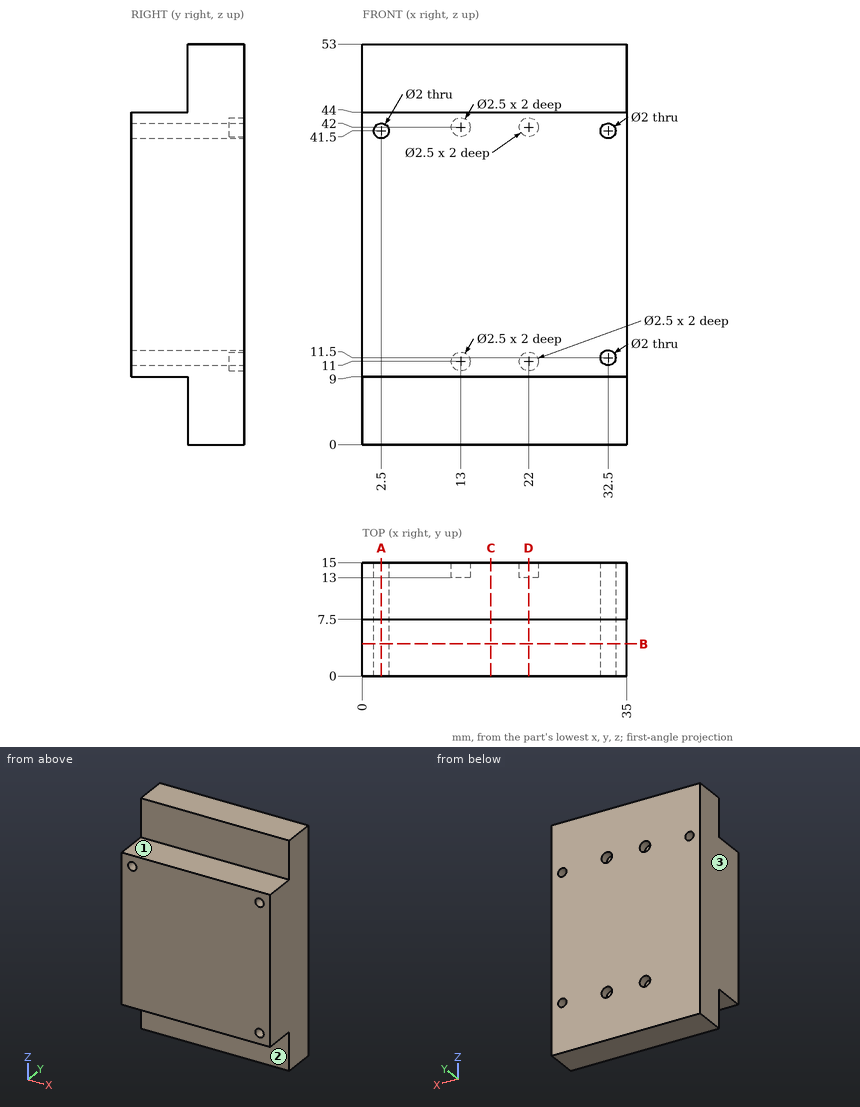
For this review, use the dimensioned drawing (mm, ordinates from the lowest corner) and the shaded views. A direction names the side the tool comes from. Give positions to 0.01 mm unless a question says otherwise; leave off trailing zeros. Write each loop counter-clockwise with the first axis right and the second up, starting at its lowest first coordinate (ties: lowest second). Pieces come first, ordered by that corner, then holes.
(1) Consider section A-A, the plane x = 2.5. Give the boundary of the cut face in (y, z), and give its area (3 significant figures).
(2) Consider section C-C, the plane x = 17. Give the boundary of the cut face in (y, z).
(3) Tool access review of the marked faces 1, 2 and 3: name each direction out of +Z, -Z, +X, -X, +Y, -Y from which nothing blocks a thin tool from reaching the whole face with its end or side.
(4) Consider section B-B, the plane y = 4.25. Give the boundary of the cut face in (x, z).
(5) To check wall thickness, follow L1, parallel to Z at x = 32.5, y = 3.75; L2, parallel to Z at x = 22, y = 14; L3, parallel to X at y = 14.5, z = 42. State the ranges of each line that lie inside material, in increasing order.
(6) Consider section D-D, the plane x = 22. Give the boundary of the cut face in (y, z).
(7) For P1, Ø0.8, axis at x = 12.5, z = 41.5, coming from the +Y side; P2, Ø4, axis at x = 14.5, y = 3.5, coming from the -Z side; P3, Ø8, axis at x = 9, y = 2, coming from the +Z side, all flat-tipped, find the tip position at first contact; note any pin that passes through.
Returned:
1. outline: (0, 9) - (7.5, 9) - (7.5, 0) - (15, 0) - (15, 40.5) - (0, 40.5) - close; (0, 42.5) - (15, 42.5) - (15, 53) - (7.5, 53) - (7.5, 44) - (0, 44) - close
1. area: 630 mm2
2. outline: (0, 9) - (7.5, 9) - (7.5, 0) - (15, 0) - (15, 53) - (7.5, 53) - (7.5, 44) - (0, 44) - close
3. face 1: +Z, +X, -X, -Y
3. face 2: -Z, +X, -X, -Y
3. face 3: +Z, -Z, -X, +Y, -Y
4. outline: (0, 9) - (35, 9) - (35, 44) - (0, 44) - close; hole circle Ø2 at (2.5, 41.5); hole circle Ø2 at (32.5, 11.5); hole circle Ø2 at (32.5, 41.5)
5. L1: z = 9 to 10.5, 12.5 to 40.5, 42.5 to 44
5. L2: z = 0 to 9.75, 12.25 to 40.75, 43.25 to 53
5. L3: x = 0 to 1.63, 3.37 to 11.75, 14.25 to 20.75, 23.25 to 31.63, 33.37 to 35
6. outline: (0, 9) - (7.5, 9) - (7.5, 0) - (15, 0) - (15, 9.75) - (13, 9.75) - (13, 12.25) - (15, 12.25) - (15, 40.75) - (13, 40.75) - (13, 43.25) - (15, 43.25) - (15, 53) - (7.5, 53) - (7.5, 44) - (0, 44) - close
7. P1: stops at y = 13
7. P2: stops at z = 9
7. P3: stops at z = 44
